Verification items for the finished model (mm, model axes). A direction names the side the tool comes from. Round coordinates to 2 decimals unless told otherwise and drop trailing zeros. Write each loop counter-clockwise with the first axis right and the second up, starting at its lowest first coordinate (ties: lowest second). Pieces come first, ordered by that corner, then holes. Notation, with made-up numbers: (31, -14) - (35, -14) arc R13 cw to (35, -9) - close; hole circle Ø11 at (-37, 41.5). An arc over 180 degrees is marked (long way). Answer as a JSON object with one key per item and string values.
```python
from build123d import *

# Parameters (mm, degrees)
SKETCH1_R           = 4.25
SKETCH1_R_2         = 2.75
BOSS_EXTRUDE1_DEPTH = 3.175


with BuildPart() as part:
    # Sketch1 → Boss-Extrude1 (new body)
    with BuildSketch(Plane(origin=(0, 0, 0), x_dir=(1, 0, 0), z_dir=(0, 1, 0))):
        with BuildLine():
            Line((-1.428652306, 7.871400929), (30.290003092, 13.628308828))
            ThreePointArc((30.290003092, 13.628308828), (37.048664607, 14.543961024), (43.8622, 14.85))
            Line((43.8622, 14.85), (98.8622, 14.85))
            ThreePointArc((98.8622, 14.85), (102.397733906, 13.385533906), (103.8622, 9.85))
            Line((103.8622, 9.85), (103.8622, 3.85))
            ThreePointArc((103.8622, 3.85), (102.397733906, 0.314466094), (98.8622, -1.15))
            Line((98.8622, -1.15), (43.8622, -1.15))
            ThreePointArc((43.8622, -1.15), (38.483093111, -1.391609718), (33.147307705, -2.114493031))
            Line((33.147307705, -2.114493031), (1.428652306, -7.871400929))
            ThreePointArc((1.428652306, -7.871400929), (-7.871400929, -1.428652306), (-1.428652306, 7.871400929))
        make_face()
        with Locations(Location((0, 0, 0), (0, 0, 270))):
            Circle(SKETCH1_R, mode=Mode.SUBTRACT)
        with Locations(Location((98.8622, 6.85, 0), (0, 0, 270))):
            Circle(SKETCH1_R_2, mode=Mode.SUBTRACT)
    extrude(amount=BOSS_EXTRUDE1_DEPTH)


solid = part.part
```
1. Cross-section at A-A (y = 0.8). Record the boundary of the cut face in (x, z), plus the area to 3 significant figures.
Completed:
{"outline": "(-1.43, -7.87) - (30.29, -13.63) arc R76 ccw to (43.86, -14.85) - (98.86, -14.85) arc R5 ccw to (103.86, -9.85) - (103.86, -3.85) arc R5 ccw to (98.86, 1.15) - (43.86, 1.15) arc R60 cw to (33.15, 2.11) - (1.43, 7.87) arc R8 ccw to start; hole circle Ø8.5 at (0, 0); hole circle Ø5.5 at (98.86, -6.85)", "area": "1,680 mm^2"}
2. Material ranges on probe 1 along Z at (x, y) = (58.5, 0.8); probe 2 along X at (y, z) = (0.75, 0); probe 3 along Z at (x, y) = (98, 0.35), recorded low to high. Write a range as from..to.
Completed:
{"probe 1": "z = -14.85..1.15", "probe 2": "x = -8..-4.25, 4.25..102.05", "probe 3": "z = -14.85..-9.46, -4.24..1.15"}
3. Mould release check, pull along X, two halves, no side actions. Record for faces 1 (the face through (38.558, 1.565, 1.385)), 2 (the face through (4.214, 1.565, -0.553)), 3 (the face through (49, 3.175, -6)): released by +X, released by -X, zero draft, split by the parting line, or undercut.
Completed:
{"face 1": "released by +X", "face 2": "undercut", "face 3": "zero draft"}
4. Go/stop test with a flat-tipped pin: pin 1 (1 mm diameter, centred on x = 59, y = 2, fed in from +Z). Record where the tip stops, or that it passes through.
Completed:
{"pin 1": "stops at z = 1.15"}
5. Access from +Z, -Z, +X, -X, +Y, -Y to the whole of each face (thin tool, end or side, straight path). Record for faces 4 (the face through (72, 2, 1.15)), 5 (the face through (103.862, 2, -7)).
Completed:
{"face 4": "+Z, +X, +Y, -Y", "face 5": "+Z, -Z, +X, +Y, -Y"}
6. Cross-section at D-D (x = 72). Record the boundary of the cut face in (y, z) (3 decimals), plus the area to 3 significant figures.
Completed:
{"outline": "(0, -14.85) - (3.175, -14.85) - (3.175, 1.15) - (0, 1.15) - close", "area": "50.8 mm^2"}
7. Cross-section at B-B (z = 0). Record the boundary of the cut face in (x, y) (3 decimals), plus the area to 3 significant figures.
Completed:
{"outline": "(-8, 0) - (-4.25, 0) - (-4.25, 3.175) - (-8, 3.175) - close; (4.25, 0) - (102.052, 0) - (102.052, 3.175) - (4.25, 3.175) - close", "area": "322 mm^2"}
8. Cross-section at C-C (x = 0). Record the boundary of the cut face in (y, z) (3 decimals), plus the area to 3 significant figures.
Completed:
{"outline": "(0, -8.131) - (3.175, -8.131) - (3.175, -4.25) - (0, -4.25) - close; (0, 4.25) - (3.175, 4.25) - (3.175, 8) - (0, 8) - close", "area": "24.2 mm^2"}
